Can you work these out from the model? Positions are in its coordinate system, mm. A direction names the side the tool comes from. Coordinates: 2 decimals unless noted, no trailing zeros. Write each loop counter-clockwise with the first axis right and the second up, starting at its lowest first coordinate (ties: lowest second). Pieces come first, ordered by that corner, then holes. Notation, with made-up numbers: (58.5, 80.25) -> (105.5, 80.25) arc R14 cw to (105.5, 88.25) -> close; hole circle Ø3 at (71, -22.75). An arc over 180 degrees is marked (long way). Use one line per item in the form item = value.
```python
from build123d import *

# Parameters (mm, degrees)
F0_W     = 200
F0_H     = 100
F1_DEPTH = 300
F2_R     = 32.658895
F3_DEPTH = 20.32


with BuildPart() as f1:
    # F0 (on Top) → F1 (new body)
    with BuildSketch(Plane.XY):
        Rectangle(F0_W, F0_H)
    extrude(amount=-F1_DEPTH)

    # F2 (on face) → F3 (cut)
    with BuildSketch(Plane.XZ.offset(50)):
        with Locations((0, -158.981949)):
            Circle(F2_R)
    extrude(amount=-F3_DEPTH, mode=Mode.SUBTRACT)


solid = f1.part
```
Q1. Suppose I cut it at A-A (x = 0). Write out the boundary of the cut face in (y, z), then the cut area to 3 significant figures.
Return value:
outline = (-50, -300) -> (50, -300) -> (50, 0) -> (-50, 0) -> (-50, -126.32) -> (-29.68, -126.32) -> (-29.68, -191.64) -> (-50, -191.64) -> close
area = 28,700 mm2
Q2. Will this pin go through, and if not, where does the flat tip stop? pin 1 (19.5 mm diameter, centred on x = -8, z = -155.5, fed in from -Y).
Return value:
pin_1 = -29.68
Q3. For faces 4 (the flat face through (100, -1, -148)), 5 (the cylindrical face through (31.15, -39.98, -149.17)), which set-ups out of +Z, -Z, +X, -X, +Y, -Y let a thin tool reach every point of the face, with its end or its side?
Return value:
face_4 = +Z, -Z, +X, +Y, -Y
face_5 = -Y
Q4. If I drill on line 1 (Z direction, x = 0, y = -42.75); line 2 (Z direction, x = 28.5, y = -44.5); line 3 (X direction, y = -32, z = -136), over which ranges is the centre line in solid material (lowest first)? Write a range as from..to.
Return value:
line_1 = -300..-191.64, -126.32..0
line_2 = -300..-174.93, -143.03..0
line_3 = -100..-23.2, 23.2..100
Q5. Suppose I cut it at B-B (x = 26). Write out the boundary of the cut face in (y, z), then the cut area to 3 significant figures.
Return value:
outline = (-50, -300) -> (50, -300) -> (50, 0) -> (-50, 0) -> (-50, -139.22) -> (-29.68, -139.22) -> (-29.68, -178.75) -> (-50, -178.75) -> close
area = 29,200 mm2
Q6. Thinking about a two-plate mould opening in Z: for faces 1 (the flat face through (0, -29.68, -159)), 2 (the flat face through (-1, 1, 0)), 3 (the flat face through (-1, 50, -148)), which applies, released by +Z, released by -Z, zero draft, split by the parting line, or undercut?
Return value:
face_1 = undercut
face_2 = released by +Z
face_3 = zero draft
